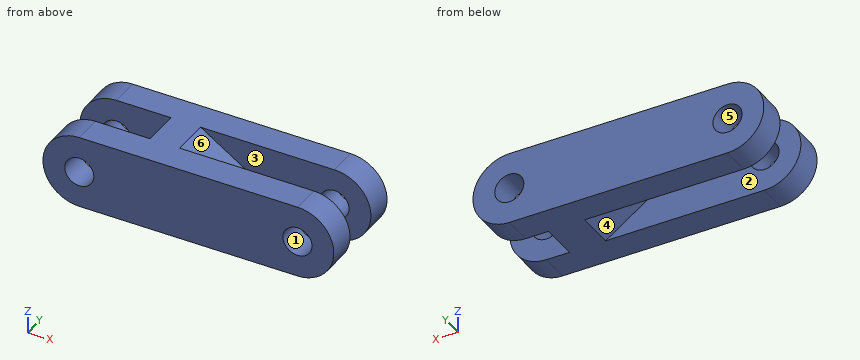
Solid Edge part; units mm, degrees
sketch "Sketch1" plane through (0, 0, 0) normal (0, -1, 0) x (1, 0, 0)
  line L0 (-10.3745, 32.1787) -> (19.6255, 32.1787)
  arc A0 (19.6255, 32.1787) -> (24.6255, 37.1787) centre (19.6255, 37.1787) ccw
  arc A1 (19.6255, 42.1787) -> (24.6255, 37.1787) centre (19.6255, 37.1787) cw
  line L1 (19.6255, 42.1787) -> (-10.3745, 42.1787)
  arc A2 (-10.3745, 42.1787) -> (-15.3745, 37.1787) centre (-10.3745, 37.1787) ccw
  arc A3 (-15.3745, 37.1787) -> (-10.3745, 32.1787) centre (-10.3745, 37.1787) ccw
extrude "Protrusion1" add sketch "Sketch1" along normal blind 13
hole "Bohrung_1" at (-10.3745, 0, 37.1787) direction (0, -1, 0) diameter 4 end through all
hole "Hole1" at (19.6255, 0, 37.1787) direction (0, -1, 0) diameter 4 end through all
sketch "Sketch2" plane through (4.6255, -6.5, 37.1787) normal (0, 1, 0) x (1, 0, 0)
  line L0 (-3.4203, -5) -> (11.829, 5)
  line L1 (11.829, 5) -> (15, 5)
  arc A0 (15, 5) -> (15, -5) centre (15, 0) cw
  line L2 (15, -5) -> (-3.4203, -5)
  line L3 (-15, 5) -> (6.8551, 5)
  line L4 (-7.4956, -5) -> (6.8551, 5)
  line L5 (-7.4956, -5) -> (-15, -5)
  arc A1 (-15, -5) -> (-15, 5) centre (-15, 0) cw
extrude "Extrusionsausschnitt_2" cut sketch "Sketch2" along normal mid plane 5.1
Input: part model. Units: mm. Frame: model coordinates. Face numbers are marked on the shaded views. A direction names the side the tool comes from. Give positions to 0.01 mm unless a question says otherwise; leave off trailing zeros. Order: outer loops, then holes, each group sorted by start corner. A loop starts at its lowest first (then second) coordinate and runs counter-clockwise, first axis right, second up. Notation, with made-up numbers: (58, 12.5) -> (90, 12.5) arc R28 cw to (90, 37.5) -> close; hole circle Ø4 at (1, 40.5). An arc over 180 degrees is marked (long way). Write each question's results on one line, items separated by ' | '. Start each with the question number.
Item 1: Set-up query: the marked faces 1, 2 and 3. Return all of +Z, -Z, +X, -X, +Y, -Y with unobstructed straight access to the full face (end or side cutting, diameter ignored); none if empty.
Item 2: Line query: line 1 (Y direction, x = -5, z = 38); line 2 (X direction, y = -3.25, z = 36); line 3 (X direction, y = -10.75, z = 39). Output: solid intervals per line, ascending.
Item 3: Cut plane A-A on x = -8. Return the cut outline in (y, z), then the cut area to 3 significant figures.
Item 4: Cut plane C-C on y = -11.75. Return the cut outline in (x, z).
Item 5: Contact query for flat-ended pins moving along their axis: P1, Ø3.5, axis at x = 19.63, z = 37.18, coming from the +Y side; P2, Ø1, axis at y = -6.5, z = 37, coming from the -X side. Output: stop coordinate, or through.
Item 6: Mould query, pull axis Z, two halves, no side actions, for the marked faces 4, 5 and 6. Classes: pulls with the +Z half, pulls with the -Z half, needs draft (parallel to the pull), parting line crosses it, or undercut.
Item 7: Cut plane B-B on z = 36.25. Return the cut outline in (x, y), then the cut area to 3 significant figures.
Item 8: Cut plane D-D on x = 18.5. Return the cut outline in (y, z).
Established:
1) face 1: +Y, -Y | face 2: -Z, -X | face 3: +Z, +X
2) line 1: -13 to -9.05, -3.95 to 0 | line 2: -15.23 to -11.99, -8.76 to 18.01, 21.24 to 24.48 | line 3: -15.03 to -11.2, -9.55 to 18.8, 20.45 to 24.28
3) outline: (-13, 32.18) -> (-9.05, 32.18) -> (-9.05, 42.18) -> (-13, 42.18) -> close; (-3.95, 32.18) -> (0, 32.18) -> (0, 42.18) -> (-3.95, 42.18) -> close | area: 79.0 mm^2
4) outline: (-10.37, 32.18) -> (19.63, 32.18) arc R5 ccw to (19.63, 42.18) -> (-10.37, 42.18) arc R5 ccw to start; hole circle Ø4 at (-10.37, 37.18); hole circle Ø4 at (19.63, 37.18)
5) P1: through | P2: x = 3.84
6) face 4: pulls with the -Z half | face 5: undercut | face 6: pulls with the +Z half
7) outline: (-15.29, -13) -> (-12.15, -13) -> (-12.15, -9.05) -> (-15.29, -9.05) -> close; (-15.29, -3.95) -> (-12.15, -3.95) -> (-12.15, 0) -> (-15.29, 0) -> close; (-8.6, -13) -> (17.85, -13) -> (17.85, -9.05) -> (10.25, -9.05) -> (10.25, -3.95) -> (17.85, -3.95) -> (17.85, 0) -> (-8.6, 0) -> (-8.6, -3.95) -> (5.64, -3.95) -> (5.64, -9.05) -> (-8.6, -9.05) -> close; (21.4, -13) -> (24.54, -13) -> (24.54, -9.05) -> (21.4, -9.05) -> close; (21.4, -3.95) -> (24.54, -3.95) -> (24.54, 0) -> (21.4, 0) -> close | area: 282 mm^2
8) outline: (-13, 32.18) -> (-9.05, 32.18) -> (-9.05, 35.53) -> (-13, 35.53) -> close; (-13, 38.83) -> (-9.05, 38.83) -> (-9.05, 42.18) -> (-13, 42.18) -> close; (-3.95, 32.18) -> (0, 32.18) -> (0, 35.53) -> (-3.95, 35.53) -> close; (-3.95, 38.83) -> (0, 38.83) -> (0, 42.18) -> (-3.95, 42.18) -> close
